```python
from build123d import *

# Parameters (mm, degrees)
F3_DEPTH   = 2487.787
F4_R       = 6.5
F5_DEPTH   = 8
F3_FACE2_W = 2487.787
F3_FACE2_H = 60
F3_FACE2_R = 6.5
F7_DEPTH   = 8.001
F6_R       = 6.5
F8_DEPTH   = 8


with BuildPart() as f3:
    # F2 (on Right) → F3 (new body)
    with BuildSketch(Plane.YZ):
        with BuildLine():
            Line((-60, 0), (0, 0))
            Line((0, 0), (0, 8))
            Line((0, 8), (-43, 8))
            ThreePointArc((-43, 8), (-51.4852813742, 11.5147186258), (-55, 20))
            Line((-55, 20), (-55, 100))
            ThreePointArc((-55, 100), (-51.4852813742, 108.4852813742), (-43, 112))
            Line((-43, 112), (0, 112))
            Line((0, 112), (0, 120))
            Line((0, 120), (-60, 120))
            Line((-60, 120), (-60, 0))
        make_face()
    extrude(amount=-F3_DEPTH)

    # F4 (on face) → F5 (cut, through all)
    with BuildSketch(Plane.XY.offset(8)):
        with Locations((-2273.377, -20)):
            Circle(F4_R)
        with Locations((-2433.377, -20)):
            Circle(F4_R)
    extrude(amount=-F5_DEPTH, mode=Mode.SUBTRACT)

    # F4 (on face) + F3_face2 (on face) → F7 (cut, through all)
    with BuildSketch(Plane.XY.offset(8)):
        with Locations((-20, -20)):
            Circle(F4_R)
        with Locations((-180, -20)):
            Circle(F4_R)
        with Locations((-2433.377, -20)):
            Circle(F4_R)
        with Locations((-2273.377, -20)):
            Circle(F4_R)
    with BuildSketch(Plane(origin=(-1241.9168214726, -30.0178162048, 0), x_dir=(1, 0, 0), z_dir=(0, 0, -1))):
        with Locations((-1.9766785274, -0.0178162048)):
            Rectangle(F3_FACE2_W, F3_FACE2_H)
        with Locations((-1191.4601785274, -10.0178162048)):
            Circle(F3_FACE2_R, mode=Mode.SUBTRACT)
        with Locations((-1031.4601785274, -10.0178162048)):
            Circle(F3_FACE2_R, mode=Mode.SUBTRACT)
    extrude(amount=-F7_DEPTH, dir=(0, 0, 1), mode=Mode.SUBTRACT)

    # F6 (on face) → F8 (cut, through all)
    with BuildSketch(Plane.XY.offset(120)):
        with Locations((-52, -20)):
            Circle(F6_R)
        with Locations((-12, -20)):
            Circle(F6_R)
        with Locations((-1052, -20)):
            Circle(F6_R)
        with Locations((-1092, -20)):
            Circle(F6_R)
        with Locations((-2307.787, -20)):
            Circle(F6_R)
        with Locations((-2467.787, -20)):
            Circle(F6_R)
    extrude(amount=-F8_DEPTH, mode=Mode.SUBTRACT)


solid = f3.part
```
The listing builds one solid part. Answer for the finished solid, in the listing's coordinates (mm). A direction names the side the tool comes from. Round coordinates to 2 decimals unless told otherwise and drop trailing zeros. Write each loop counter-clockwise with the first axis right and the second up, starting at its lowest first coordinate (ties: lowest second). Pieces come first, ordered by that corner, then holes. Notation, with made-up numbers: (-6.5, 77) -> (14.5, 77) arc R23 cw to (14.5, 89) -> close; hole circle Ø1 at (41.5, -38.75). An arc over 180 degrees is marked (long way). Answer as a JSON object with one key per item and string values. Group by question number.
Q1. Straight lines are drawn through the part: line 1 along Y through (x, z) = (-20, 2.5); line 2 along Z through (x, y) = (-1776, -12); line 3 along Z through (x, y) = (-479, -45.5). For each, find the intervals that lie inside material, in ascending order.
Q2. Which of the six approach directions +Z, -Z, +X, -X, +Y, -Y give full straight-line access (tool end or side, diameter ignored) to faces 1 (the face through (-1226, -60, 61)), 2 (the face through (-1226, -22, 112))?
Q3. Section B-B (z = 52.5) is taken. Write down the section's boundary in (x, y).
Q4. Each of these flat-tipped pins is pushed along its axis until it touches: pin 1 Ø10.5 at (x, y) = (-2433.377, -20) entering from -Z; pin 2 Ø3 at (x, z) = (-1185, 85) entering from +Y. Where does it stop, or does it pass through?
Q5. Section A-A (x = -1399) is taken. Write down the section's boundary in (y, z).
Check values:
{
 "1": {"line 1": "-60 to -26.5, -13.5 to 0", "line 2": "0 to 8, 112 to 120", "line 3": "0 to 8.26, 111.74 to 120"},
 "2": {"face 1": "+Z, -Z, +X, -X, -Y", "face 2": "+X, -X, +Y"},
 "3": {"outline": "(-2487.79, -60) -> (0, -60) -> (0, -55) -> (-2487.79, -55) -> close"},
 "4": {"pin 1": "z = 112", "pin 2": "y = -55"},
 "5": {"outline": "(-60, 0) -> (0, 0) -> (0, 8) -> (-43, 8) arc R12 cw to (-55, 20) -> (-55, 100) arc R12 cw to (-43, 112) -> (0, 112) -> (0, 120) -> (-60, 120) -> close"}
}
